Work out the finished part from the listing and answer in its coordinate system (mm). A direction names the side the tool comes from. Round coordinates to 2 decimals unless told otherwise and drop trailing zeros. Order: outer loops, then holes, each group sorted by start corner. A loop starts at its lowest first (then second) coordinate and runs counter-clockwise, first axis right, second up. Notation, with made-up numbers: M 16,11 L 26,11 A15 cw 26,17 Z; hole C 19,51.25 d9. An arc over 180 degrees is marked long. Return JSON: item names as keys, results as strings.
from build123d import *

# Parameters (mm, degrees)
SKICA1_W                      = 43.4
SKICA1_H                      = 20.8
SKICA1_R                      = 1.55
P_IDAT_VYSUNUT_M1_DEPTH       = 1.2
SKICA3_W                      = 12.1
SKICA3_H                      = 12.1
P_IDAT_VYSUNUT_M2_DEPTH       = 7.4
ZAOBLIT1_R                    = 3
SKICA4_W                      = 9.6
SKICA4_H                      = 4.5
P_IDAT_VYSUNUT_M3_DEPTH       = 10.4
SKICA5_R                      = 1.15
P_IDAT_VYSUNUT_M4_DEPTH       = 1.8
SKICA6_W                      = 8.3
SKICA6_H                      = 8.3
SKICA6_R                      = 4
P_IDAT_VYSUNUT_M5_DEPTH       = 1.5
SKICA6_2_R                    = 4
P_IDAT_VYSUNUT_M6_DEPTH       = 10.7
ZAOBLIT2_R                    = 0.5
SKICA7_W                      = 9.3
SKICA7_H                      = 8.5
P_IDAT_VYSUNUT_M7_DEPTH       = 4.5
SKICA7_3_W                    = 9.3
SKICA7_3_H                    = 1.3
P_IDAT_VYSUNUT_M8_DEPTH       = 1.4
SKICA7_4_W                    = 8
SKICA7_4_H                    = 3.4
P_IDAT_VYSUNUT_M9_DEPTH       = 1.25
SKICA7_5_W                    = 8
SKICA7_5_H                    = 1.5
P_IDAT_VYSUNUT_M10_DEPTH      = 3.5
ZKOSEN_1_SIZE                 = 2
ZKOSEN_1_SIZE2                = 0.727940469
ZAOBLIT3_R                    = 1
ZAOBLIT4_R                    = 1
ZAOBLIT5_R                    = 1
SKICA8_W                      = 5.6
SKICA8_H                      = 0.8
P_IDAT_VYSUNUT_M11_DEPTH      = 0.4
SKICA8_3_W                    = 4.1
SKICA8_3_H                    = 2.6
P_IDAT_VYSUNUT_M12_DEPTH      = 2.9
SKICA9_W                      = 1.2
SKICA9_H                      = 1.8
SKICA9_H_2                    = 2.1
P_IDAT_VYSUNUT_M13_DEPTH      = 1
SKICA10_W                     = 1.2
SKICA10_H                     = 2.1
P_IDAT_VYSUNUT_M14_DEPTH      = 0.8
P_IDAT_VYSUNUT_M15_DEPTH      = 0.1
P_IDAT_VYSUNUT_M15_DEPTH_BACK = 1.3
SKICA11_W                     = 3
SKICA11_H                     = 3
SKICA11_R                     = 0.75
SKICA11_2_R                   = 0.75
ODEBRAT_VYSUNUT_M1_DEPTH      = 27.979436614
SKICA12_W                     = 3.658871704
SKICA12_H                     = 0.6
ODEBRAT_VYSUNUT_M2_DEPTH      = 0.5
SKICA13_W                     = 1.5
SKICA13_H                     = 1.5
P_IDAT_VYSUNUT_M16_DEPTH      = 1.1


with BuildPart() as part:
    # Skica1 → Přidat vysunutím1 (new body)
    with BuildSketch(Plane.XY):
        Rectangle(SKICA1_W, SKICA1_H)
        with Locations((-15.05, 7.85)):
            Circle(SKICA1_R, mode=Mode.SUBTRACT)
        with Locations((15.45, -8.05)):
            Circle(SKICA1_R, mode=Mode.SUBTRACT)
    extrude(amount=P_IDAT_VYSUNUT_M1_DEPTH)

    # Skica3 → Přidat vysunutím2 (add)
    with BuildSketch(Plane.XY.offset(1.2)):
        with Locations((-5.95, -2.55)):
            Rectangle(SKICA3_W, SKICA3_H)
    extrude(amount=P_IDAT_VYSUNUT_M2_DEPTH)

    # Zaoblit1
    zaoblit1_edges = [part.edges().sort_by_distance(p)[0] for p in [
        (0.1, -8.6, 4.9),
        (0.1, 3.5, 4.9),
        (-12, 3.5, 4.9),
        (-12, -8.6, 4.9),
    ]]
    fillet(zaoblit1_edges, radius=ZAOBLIT1_R)

    # Skica4 → Přidat vysunutím3 (add)
    with BuildSketch(Plane.XY.offset(1.2)):
        with Locations((-6.1, 7.15)):
            Rectangle(SKICA4_W, SKICA4_H)
    extrude(amount=P_IDAT_VYSUNUT_M3_DEPTH)

    # Skica5 → Přidat vysunutím4 (add)
    with BuildSketch(Plane.XY.offset(11.6)):
        with Locations(Location((-9.75, 8.25, 0), (0, 0, 180))):
            Circle(SKICA5_R)
    extrude(amount=P_IDAT_VYSUNUT_M4_DEPTH)

    # Skica6 → Přidat vysunutím5 (add)
    # profile 1 of 2: a face of its own
    with BuildSketch(Plane.XY.offset(1.2)):
        with Locations((-16.65, -0.25)):
            Rectangle(SKICA6_W, SKICA6_H)
        with Locations((-16.65, -0.25)):
            Circle(SKICA6_R, mode=Mode.SUBTRACT)
    # profile 2 of 2: a face of its own
    with BuildSketch(Plane.XY.offset(1.2)):
        with Locations((16.55, -0.25)):
            Rectangle(SKICA6_W, SKICA6_H)
        with Locations((16.55, -0.25)):
            Circle(SKICA6_R, mode=Mode.SUBTRACT)
    extrude(amount=P_IDAT_VYSUNUT_M5_DEPTH)

    # Skica6<2> → Přidat vysunutím6 (add)
    with BuildSketch(Plane.XY.offset(1.2)):
        with Locations((-16.65, -0.25)):
            Circle(SKICA6_2_R)
        with Locations((16.55, -0.25)):
            Circle(SKICA6_2_R)
    extrude(amount=P_IDAT_VYSUNUT_M6_DEPTH)

    # Zaoblit2
    zaoblit2_edges = [part.edges().sort_by_distance(p)[0] for p in [
        (-20.65, -0.25, 11.9),
        (12.55, -0.25, 11.9),
    ]]
    fillet(zaoblit2_edges, radius=ZAOBLIT2_R)

    # Skica7 → Přidat vysunutím7 (add)
    with BuildSketch(Plane.XY.offset(1.2)):
        with Locations((6.85, -4.25)):
            Rectangle(SKICA7_W, SKICA7_H)
    extrude(amount=P_IDAT_VYSUNUT_M7_DEPTH)

    # Skica7<3> → Přidat vysunutím8 (add)
    with BuildSketch(Plane.XY.offset(1.2)):
        with Locations((6.85, -9.15)):
            Rectangle(SKICA7_3_W, SKICA7_3_H)
    extrude(amount=P_IDAT_VYSUNUT_M8_DEPTH)

    # Skica7<4> → Přidat vysunutím9 (add)
    with BuildSketch(Plane.XY.offset(1.2)):
        with Locations((6.85, 3.2)):
            Rectangle(SKICA7_4_W, SKICA7_4_H)
    extrude(amount=P_IDAT_VYSUNUT_M9_DEPTH)

    # Skica7<5> → Přidat vysunutím10 (add)
    with BuildSketch(Plane.XY.offset(1.2)):
        with Locations((6.85, 0.75)):
            Rectangle(SKICA7_5_W, SKICA7_5_H)
    extrude(amount=P_IDAT_VYSUNUT_M10_DEPTH)

    # Zkosení1
    zkosen_1_edges = [part.edges().sort_by_distance(p)[0] for p in [
        (6.85, 1.5, 2.45),
    ]]
    zkosen_1_side = [part.faces().sort_by_distance(p)[0] for p in [
        (6.85, 1.5, 3.575),
    ]]
    chamfer(zkosen_1_edges, length=ZKOSEN_1_SIZE, length2=ZKOSEN_1_SIZE2, reference=zkosen_1_side[0])

    # Zaoblit3
    # the kernel refuses this fillet: 1 mm, written as the material it takes off along each edge
    with BuildSketch(Plane(origin=(12.503594569, 1.5, 4.7), x_dir=(0, 0, -1), z_dir=(-1, 0, 0))) as zaoblit3_piece_1:
        with BuildLine():
            CenterArc((1, 0.661437828), ZAOBLIT3_R, 180, 41.409622109)
            Line((0, 0.661437828), (-0.02, 0.661437828))
            Line((-0.02, 0.661437828), (-0.02, 0))
            Line((-0.02, 0), (0, -0.02))
            ThreePointArc((0, -0.02), (0.125, -0.02), (0.235, -0.013228757))
            Line((0.235, -0.013228757), (0.25, 0))
        make_face()
    extrude(amount=11.307189139, mode=Mode.SUBTRACT)

    # Zaoblit4
    # the kernel refuses this fillet: 1 mm, written as the material it takes off along each edge
    with BuildSketch(Plane(origin=(0.775606123, 1.5, 4.45), x_dir=(0, -0.953531662347256, 0.30129282915675026), z_dir=(1, 0, 0))) as zaoblit4_piece_1:
        with BuildLine():
            CenterArc((0.528464722, 0.953531662), ZAOBLIT4_R, 217.535269991, 70)
            Line((-0.264513729, 0.344281978), (-0.343811574, 0.28335701))
            Line((-0.343811574, 0.28335701), (-0.079297845, -0.060924968))
            Line((-0.079297845, -0.060924968), (-0.040473229, -0.091443522))
            ThreePointArc((-0.040473229, -0.091443522), (0.736154402, -0.134449607), (0.859886834, -0.095353166))
            Line((0.859886834, -0.095353166), (0.829757551, 0))
        make_face()
    extrude(amount=10.074393877, mode=Mode.SUBTRACT)

    # Zaoblit5
    zaoblit5_edges = [part.edges().sort_by_distance(p)[0] for p in [
        (6.85, 2.227940469, 2.45),
    ]]
    fillet(zaoblit5_edges, radius=ZAOBLIT5_R)

    # Skica8 → Přidat vysunutím11 (add)
    with BuildSketch(Plane.XY.offset(1.2)):
        with Locations((9.05, 8)):
            Rectangle(SKICA8_W, SKICA8_H)
    extrude(amount=P_IDAT_VYSUNUT_M11_DEPTH)

    # Skica8<3> → Přidat vysunutím12 (add)
    with BuildSketch(Plane.XY.offset(1.2)):
        with Locations((9.05, 8)):
            Rectangle(SKICA8_3_W, SKICA8_3_H)
    extrude(amount=P_IDAT_VYSUNUT_M12_DEPTH)

    # Skica9 → Přidat vysunutím13 (add)
    with BuildSketch(Plane.XY.offset(1.2)):
        with Locations((1.2, 3.8)):
            Rectangle(SKICA9_W, SKICA9_H)
        with Locations((1.2, 7.85)):
            Rectangle(SKICA9_W, SKICA9_H_2)
    extrude(amount=P_IDAT_VYSUNUT_M13_DEPTH)

    # Skica10 → Přidat vysunutím14 (add)
    with BuildSketch(Plane.XY.offset(1.2)):
        with Locations((13.3, 6.65)):
            Rectangle(SKICA10_W, SKICA10_H)
    extrude(amount=P_IDAT_VYSUNUT_M14_DEPTH)

    # Skica11 → Přidat vysunutím15 (add, two sides: drawn at the far end of the back side and taken through both)
    # profile 1 of 4: a face of its own
    with BuildSketch(Plane.XY.offset(1.2).offset(-P_IDAT_VYSUNUT_M15_DEPTH_BACK)):
        with Locations((19.95, -8.75)):
            Rectangle(SKICA11_W, SKICA11_H)
        with Locations((19.95, -8.75)):
            Circle(SKICA11_R, mode=Mode.SUBTRACT)
    # profile 2 of 4: a face of its own
    with BuildSketch(Plane.XY.offset(1.2).offset(-P_IDAT_VYSUNUT_M15_DEPTH_BACK)):
        with Locations((19.95, 8.75)):
            Rectangle(SKICA11_W, SKICA11_H)
        with Locations((19.95, 8.75)):
            Circle(SKICA11_R, mode=Mode.SUBTRACT)
    # profile 3 of 4: a face of its own
    with BuildSketch(Plane.XY.offset(1.2).offset(-P_IDAT_VYSUNUT_M15_DEPTH_BACK)):
        with Locations((-20.05, -8.75)):
            Rectangle(SKICA11_W, SKICA11_H)
        with Locations((-20.05, -8.75)):
            Circle(SKICA11_R, mode=Mode.SUBTRACT)
    # profile 4 of 4: a face of its own
    with BuildSketch(Plane.XY.offset(1.2).offset(-P_IDAT_VYSUNUT_M15_DEPTH_BACK)):
        with Locations((-20.05, 8.75)):
            Rectangle(SKICA11_W, SKICA11_H)
        with Locations((-20.05, 8.75)):
            Circle(SKICA11_R, mode=Mode.SUBTRACT)
    extrude(amount=P_IDAT_VYSUNUT_M15_DEPTH + P_IDAT_VYSUNUT_M15_DEPTH_BACK)

    # Skica11<2> → Odebrat vysunutím1 (cut, through all)
    with BuildSketch(Plane.XY.offset(1.2)):
        with Locations((-20.05, 8.75)):
            Circle(SKICA11_2_R)
        with Locations((-20.05, -8.75)):
            Circle(SKICA11_2_R)
        with Locations((19.95, 8.75)):
            Circle(SKICA11_2_R)
        with Locations((19.95, -8.75)):
            Circle(SKICA11_2_R)
    extrude(amount=-ODEBRAT_VYSUNUT_M1_DEPTH, mode=Mode.SUBTRACT)

    # Skica12 → Odebrat vysunutím2 (cut)
    with BuildSketch(Plane.XY.offset(13.4)):
        with Locations((-9.75, 8.25)):
            Rectangle(SKICA12_W, SKICA12_H)
    extrude(amount=-ODEBRAT_VYSUNUT_M2_DEPTH, mode=Mode.SUBTRACT)

    # Skica13 → Přidat vysunutím16 (add)
    with BuildSketch(Plane(origin=(0, 0, 0), x_dir=(-1, 0, 0), z_dir=(0, 0, -1))):
        with Locations((3.85, 7.15)):
            Rectangle(SKICA13_W, SKICA13_H)
        with Locations((6.25, 7.15)):
            Rectangle(SKICA13_W, SKICA13_H)
        with Locations((8.65, 7.15)):
            Rectangle(SKICA13_W, SKICA13_H)
    extrude(amount=P_IDAT_VYSUNUT_M16_DEPTH)


solid = part.part
Item 1: Consider line 1 along X through (y, z) = (-4.25, 1.75); line 2 along Y through (x, z) = (19.95, 0.25); line 3 along Y through (x, z) = (15.45, 0.5). Determine where each line is inside the solid, lowest interval first. Write a range as [from, to].
Output:
{"line 1": "x = [-20.8, -12.5], [-12, 0.1], [2.2, 11.5], [12.4, 20.7]", "line 2": "y = [-10.4, -9.5], [-8, 8], [9.5, 10.4]", "line 3": "y = [-10.4, -9.6], [-6.5, 10.4]"}
Item 2: The mould has two halves that part along X. Classify faces 6 (the cylindrical face through (-0.8, -7.74, 4.95)), 7 (the flat face through (-6, 4.9, 6)), 8 (the cylindrical face through (-0.76, 2.6, 4.95)), 9 (the cylindrical face through (-10.847, 7.905, 12.487)): pulls with the +X half, pulls with the -X half, needs draft (parallel to the pull), parting line crosses it, or undercut.
Output:
{"face 6": "undercut", "face 7": "needs draft", "face 8": "undercut", "face 9": "parting line crosses it"}
Item 3: Which of the six approach directions +Z, -Z, +X, -X, +Y, -Y give full straight-line access (tool end or side, diameter ignored) to faces 1 (the cylindrical face through (6.9, 2.4, 2.6)), 2 (the flat face through (1, 4, 2.2)), 3 (the flat face through (-6, -2, 8.6)), 4 (the flat face through (-6, 9.4, 6)), 5 (the flat face through (19, 9, -0.1))?
Output:
{"face 1": "+Z", "face 2": "+Z, +Y, -Y", "face 3": "+Z, -Y", "face 4": "+Z, +X, -X, +Y", "face 5": "-Z, +X, +Y, -Y"}
Item 4: Each of these flat-tipped pins is pushed along its axis until it touches: pin 1 (6.5 mm diameter, centred on x = -14.5, y = -2.5, fed in from +Z); pin 2 (2 mm diameter, centred on y = -3.5, z = 2.5, fed in from +X); pin 3 (6 mm diameter, centred on x = -1, y = 1.5, fed in from -Z). Where does it stop, or does it pass through?
Output:
{"pin 1": "stops at z = 11.9", "pin 2": "stops at x = 20.7", "pin 3": "stops at z = 0"}
Item 5: Find section B-B (x = 16.55). Determine the outline of the cut face in (y, z).
Output:
{"outline": "M -10.4,0 L -9.14,0 L -9.14,1.2 L -10.4,1.2 Z; M -6.96,0 L 10.4,0 L 10.4,1.2 L 3.9,1.2 L 3.9,2.7 L 3.75,2.7 L 3.75,11.4 A0.5 ccw 3.25,11.9 L -3.75,11.9 A0.5 ccw -4.25,11.4 L -4.25,2.7 L -4.4,2.7 L -4.4,1.2 L -6.96,1.2 Z"}
Item 6: Find section A-A (x = 9). Determine the outline of the cut face in (y, z), plus the area to 3 significant figures.
Output:
{"outline": "M -10.4,0 L 10.4,0 L 10.4,1.2 L 9.3,1.2 L 9.3,4.1 L 6.7,4.1 L 6.7,1.2 L 4.9,1.2 L 4.9,2.45 L 2.93,2.45 A1 cw 1.99,3.11 L 1.65,4.04 A1 ccw 0.71,4.7 L 0,4.7 L 0,5.7 L -8.5,5.7 L -8.5,2.6 L -9.8,2.6 L -9.8,1.2 L -10.4,1.2 Z", "area": "82.8 mm^2"}
